```python
from build123d import *

# Parameters (mm, degrees)
BOSS_EXTRUDE1_START     = 92.868812
BOSS_EXTRUDE1_DEPTH     = 3.175
F_1_4_CLEARANCE_HOLE1_D = 6.7564
FILLET1_R               = 6.35


with BuildPart() as part:
    # Sketch1 → Boss-Extrude1 (new body)
    with BuildSketch(Plane(origin=(0, 0, 0), x_dir=(0, 0, -1), z_dir=(1, 0, 0)).offset(BOSS_EXTRUDE1_START)):
        with BuildLine():
            Line((-1321.740142063, 202.439766645), (-1270.940142063, 151.639766645))
            ThreePointArc((-1270.940142063, 151.639766645), (-1268.875381607, 141.259514861), (-1277.675334154, 135.379574554))
            Line((-1277.675334154, 135.379574554), (-1303.075334154, 135.379574554))
            ThreePointArc((-1303.075334154, 135.379574554), (-1309.810526245, 138.169382463), (-1312.600334154, 144.904574554))
            Line((-1312.600334154, 144.904574554), (-1312.600334154, 160.779574554))
            Line((-1312.600334154, 160.779574554), (-1328.475334154, 160.779574554))
            ThreePointArc((-1328.475334154, 160.779574554), (-1335.210526245, 163.569382463), (-1338.000334154, 170.304574554))
            Line((-1338.000334154, 170.304574554), (-1338.000334154, 195.704574554))
            ThreePointArc((-1338.000334154, 195.704574554), (-1332.120393847, 204.504527101), (-1321.740142063, 202.439766645))
        make_face()
    extrude(amount=BOSS_EXTRUDE1_DEPTH)

    # 1/4 Clearance Hole1 (through all)
    with Locations(Plane.ZY.offset(-92.868812484)):
        with Locations((1328.475334154, 195.704574554), (1328.475334154, 170.304574554), (1277.675334154, 144.904574554), (1303.075334154, 144.904574554)):
            Hole(F_1_4_CLEARANCE_HOLE1_D / 2)

    # Fillet1
    fillet1_edges = [part.edges().sort_by_distance(p)[0] for p in [
        (94.456312, 160.779574554, 1312.600334154),
    ]]
    fillet(fillet1_edges, radius=FILLET1_R)


solid = part.part
```
Check sheet for the modelled part. Datum: model origin and axes. Units: mm. A direction names the side the tool comes from. Round coordinates to 2 decimals unless told otherwise and drop trailing zeros. Write each loop counter-clockwise with the first axis right and the second up, starting at its lowest first coordinate (ties: lowest second). Pieces come first, ordered by that corner, then holes. Notation, with made-up numbers: (73, 43) -> (80, 43) arc R26 ccw to (80, 70) -> close; hole circle Ø3 at (48, 68). An arc over 180 degrees is marked (long way). One line per question, with ' | ' between items. Start each with the question number.
1. Release check for a two-part mould opening along Y. For faces 3 (the face through (94.43, 204.44, 1332.27)), 4 (the face through (94.48, 158.97, 1314.51)), 5 (the face through (94.479, 145.919, 1274.453)) record: +Y half, -Y half, draft (parallel to the pull), parting line (faces both ways), or undercut.
2. Sectioned sample at B-B, the plane z = 1300.5. Record the cut outline in (x, y), then the cut area to 3 significant figures.
3. Sectioned sample at C-C, the plane y = 197. Record the cut outline in (x, z), then the cut area to 3 significant figures.
4. Scan lines: line 1 along Y through (x, z) = (94.25, 1331); line 2 along Z through (x, y) = (95.6, 198.5); line 3 along Y through (x, z) = (93, 1330). Record each from-to range of solid material in increasing order. Write a range as from..to.
5. Set-up check for faces 1 (the face through (94.479, 145.919, 1299.853)), 2 (the face through (94, 160.78, 1324)): record each of +Z, -Z, +X, -X, +Y, -Y from which the full face is reachable in a straight line by a thin tool's end or side.
6. Sectioned sample at D-D, the plane y = 158. Record the cut outline in (x, z), then the cut area to 3 significant figures.
7. Sectioned sample at A-A, the plane x = 94.9. Record the cut outline in (y, z) (3 decimals).
8. Depth check by flat-ended pin: pin 1 (1.5 mm diameter, centred on x = 94.5, z = 1298.5, fed in from +Y); pin 2 (1 mm diameter, centred on x = 95, y = 151, fed in from +Z). Enter the tip coordinate at first touch or a pass-through.
Taken from the geometry:
1) face 3: +Y half | face 4: -Y half | face 5: undercut
2) outline: (92.87, 135.38) -> (96.04, 135.38) -> (96.04, 142.72) -> (92.87, 142.72) -> close; (92.87, 147.09) -> (96.04, 147.09) -> (96.04, 181.2) -> (92.87, 181.2) -> close | area: 132 mm^2
3) outline: (92.87, 1316.3) -> (96.04, 1316.3) -> (96.04, 1325.36) -> (92.87, 1325.36) -> close; (92.87, 1331.6) -> (96.04, 1331.6) -> (96.04, 1337.91) -> (92.87, 1337.91) -> close | area: 48.8 mm^2
4) line 1: y = 161.12..168.06, 172.55..193.46, 197.95..204.89 | line 2: z = 1317.8..1326.58, 1330.37..1337.58 | line 3: y = 160.9..167.29, 173.32..192.69, 198.72..205.11
5) face 1: +X, -X | face 2: +Z, +X, -X, -Y
6) outline: (92.87, 1277.3) -> (96.04, 1277.3) -> (96.04, 1313.7) -> (92.87, 1313.7) -> close | area: 116 mm^2
7) outline: (135.38, 1277.675) arc R9.525 ccw to (151.64, 1270.94) -> (202.44, 1321.74) arc R9.525 ccw to (195.705, 1338) -> (170.305, 1338) arc R9.525 ccw to (160.78, 1328.475) -> (160.78, 1318.95) arc R6.35 cw to (154.43, 1312.6) -> (144.905, 1312.6) arc R9.525 ccw to (135.38, 1303.075) -> close; hole circle Ø6.756 at (144.905, 1277.675); hole circle Ø6.756 at (144.905, 1303.075); hole circle Ø6.756 at (170.305, 1328.475); hole circle Ø6.756 at (195.705, 1328.475)
8) pin 1: stops at y = 179.95 | pin 2: stops at z = 1312.6
